Build history of the part. All positions in model axes, mm. A direction names the side the tool comes from. Round coordinates to 2 decimals unless told otherwise and drop trailing zeros. Order: outer loops, then holes, each group sorted by start corner. A loop starts at its lowest first (then second) coordinate and runs counter-clockwise, first axis right, second up. Notation, with made-up numbers: M 51.5,29.25 L 110.5,29.25 A31 cw 110.5,64.25 Z; hole C 81.25,16 d10. An arc over 180 degrees is marked long. Use CSV: the item, a comma, the result in double quotes.
from build123d import *

# Parameters (mm, degrees)
ESQUISSE1_R             = 6.125
BOSS_EXTRU_1_DEPTH      = 22
BOSS_EXTRU_2_DEPTH      = 15.875
BOSS_EXTRU_2_DEPTH_BACK = 15.875
BOSS_EXTRU_2_START      = -11
ESQUISSE2_R             = 1.375
ESQUISSE3_R             = 1.875
BOSS_EXTRU_3_DEPTH      = 1.5
BOSS_EXTRU_4_START      = -1.5
ESQUISSE4_R             = 1.875
BOSS_EXTRU_4_DEPTH      = 1.5
CHANFREIN1_SIZE         = 10.25
CHANFREIN1_SIZE_2       = 4.779653496
CONG_1_R                = 3.25
CONG_2_R                = 0.25


with BuildPart() as part:
    # Esquisse1 → Boss.-Extru.1 (new body)
    with BuildSketch(Plane.XY):
        Circle(ESQUISSE1_R)
    extrude(amount=BOSS_EXTRU_1_DEPTH)

    # Esquisse2 → Boss.-Extru.2 (add, two sides: drawn at the far end of the back side and taken through both)
    with BuildSketch(Plane.XY.offset(22).offset(BOSS_EXTRU_2_START - BOSS_EXTRU_2_DEPTH_BACK)):
        Circle(ESQUISSE2_R)
    extrude(amount=BOSS_EXTRU_2_DEPTH + BOSS_EXTRU_2_DEPTH_BACK)

    # Esquisse3 → Boss.-Extru.3 (add)
    with BuildSketch(Plane(origin=(0, 0, -4.875), x_dir=(-1, 0, 0), z_dir=(0, 0, -1))):
        Circle(ESQUISSE3_R)
    extrude(amount=-BOSS_EXTRU_3_DEPTH)

    # Esquisse4 → Boss.-Extru.4 (add)
    with BuildSketch(Plane.XY.offset(26.875).offset(BOSS_EXTRU_4_START)):
        with Locations(Location((0, 0, 0), (0, 0, 180))):
            Circle(ESQUISSE4_R)
    extrude(amount=BOSS_EXTRU_4_DEPTH)

    # Chanfrein1
    # the kernel refuses this chamfer: 10.25, 4.779653496 mm, written as the material it takes off along each edge
    with BuildSketch(Plane(origin=(0, 0, 22), x_dir=(1, 0, 0), z_dir=(0, -1, 0))) as chanfrein1_piece_1_section:
        Polygon((6.125, -CHANFREIN1_SIZE), (6.125 - CHANFREIN1_SIZE_2, 0), (6.125, 0), align=None)
    chanfrein1_piece_1 = revolve(axis=Axis((0, 0, 22), (0, 0, 1)), mode=Mode.PRIVATE)
    chanfrein1_piece_1 = chanfrein1_piece_1 - Plane(origin=(0, 0, 16.69695502), x_dir=(1, 0, 0), z_dir=(0, 0, -1)) * Cylinder(1.375, 41, mode=Mode.PRIVATE)
    add(chanfrein1_piece_1, mode=Mode.SUBTRACT)
    with BuildSketch(Plane(origin=(0, 0, 0), x_dir=(1, 0, 0), z_dir=(0, -1, 0))) as chanfrein1_piece_2_section:
        Polygon((6.125, CHANFREIN1_SIZE), (6.125 - CHANFREIN1_SIZE_2, 0), (6.125, 0), align=None)
    chanfrein1_piece_2 = revolve(axis=Axis((0, 0, 0), (0, 0, 1)), mode=Mode.PRIVATE)
    chanfrein1_piece_2 = chanfrein1_piece_2 - Plane(origin=(0, 0, 5.30304498), x_dir=(1, 0, 0), z_dir=(0, 0, 1)) * Cylinder(1.375, 41, mode=Mode.PRIVATE)
    add(chanfrein1_piece_2, mode=Mode.SUBTRACT)

    # Congé1
    cong_1_edges = [part.edges().sort_by_distance(p)[0] for p in [
        (-6.125, 0, 11.75),
        (-6.125, 0, 10.25),
    ]]
    fillet(cong_1_edges, radius=CONG_1_R)

    # Congé2
    cong_2_edges = [part.edges().sort_by_distance(p)[0] for p in [
        (1.875, 0, -3.375),
        (1.875, 0, -4.875),
        (1.875, 0, 25.375),
        (1.875, 0, 26.875),
    ]]
    fillet(cong_2_edges, radius=CONG_2_R)


solid = part.part
(1) Tool access for faces 1 (the face through (-1.01, -1.58, 26.12)), 2 (the face through (0, 0, 26.875)), 3 (the face through (1.873, 0.082, -4.132)): list every direction of +Z, -Z, +X, -X, +Y, -Y with a clear straight run to the whole face (end or side of a thin tool).
Answer block:
face 1,"+Z"
face 2,"+Z, +X, -X, +Y, -Y"
face 3,"-Z"
(2) Cut at A-A, the plane z = 22.5. Give the cut face in (x, y) (3 decimals), and give its area (3 significant figures).
Answer block:
outline,"C 0,0 d2.75"
area,"5.94 mm²"
(3) Drop flat-ended pins along their axis: pin 1 (2 mm diameter, centred on y = 3.5, z = 15, fed in from +X); pin 2 (1.5 mm diameter, centred on y = -3.5, z = 15.5, fed in from -X); pin 3 (1.5 mm diameter, centred on y = 0.5, z = 22.5, fed in from -X). Give the stop position or say it passes through.
Answer block:
pin 1,"stops at x = 4.08"
pin 2,"stops at x = -3.55"
pin 3,"stops at x = -1.42"
(4) Wall check: line 1 (Z direction, x = -0.5, y = 1.5) (3 decimals); line 2 (Y direction, x = -3, z = 8.5); line 3 (Z direction, x = -1.5, y = 4.75). Give the ranges that are in metal, low to high. Write a range as from..to.
Answer block:
line 1,"z = -4.875..-3.375, 0.506..21.494, 25.375..26.875"
line 2,"y = -4.38..4.38"
line 3,"z = 7.8..14.2"
